from build123d import *

# Parameters (mm, degrees)
CROQUIS1_W              = 28
CROQUIS1_H              = 48
SALIENTE_EXTRUIR1_DEPTH = 2
CROQUIS2_R              = 1.25
CORTAR_EXTRUIR1_DEPTH   = 3
CROQUIS3_W              = 15
CROQUIS3_H              = 15
SALIENTE_EXTRUIR2_DEPTH = 6


with BuildPart() as part:
    # Croquis1 → Saliente-Extruir1 (new body)
    with BuildSketch(Plane.XY):
        Rectangle(CROQUIS1_W, CROQUIS1_H)
    extrude(amount=SALIENTE_EXTRUIR1_DEPTH)

    # Croquis2 → Cortar-Extruir1 (cut, through all)
    with BuildSketch(Plane.XY.offset(2)):
        with Locations((-10, 20)):
            Circle(CROQUIS2_R)
        with Locations((10, 20)):
            Circle(CROQUIS2_R)
        with Locations((10, -20)):
            Circle(CROQUIS2_R)
        with Locations((-10, -20)):
            Circle(CROQUIS2_R)
    extrude(amount=-CORTAR_EXTRUIR1_DEPTH, mode=Mode.SUBTRACT)

    # Croquis3 → Saliente-Extruir2 (add)
    with BuildSketch(Plane.XY.offset(2)):
        with Locations((6.5, 4.293122568)):
            Rectangle(CROQUIS3_W, CROQUIS3_H)
    extrude(amount=SALIENTE_EXTRUIR2_DEPTH)


solid = part.part
Can you work these out from the model? Positions are in its coordinate system, mm. A direction names the side the tool comes from. Give positions to 0.01 mm unless a question says otherwise; leave off trailing zeros. Write each loop counter-clockwise with the first axis right and the second up, starting at its lowest first coordinate (ties: lowest second). Pieces come first, ordered by that corner, then holes. Notation, with made-up numbers: (34, 25) -> (82, 25) arc R15 ccw to (82, 29) -> close; hole circle Ø10 at (19, 7). An arc over 180 degrees is marked (long way). Answer as a JSON object with one key per item and string values. Group by question number.
Item 1: Suppose I cut it at D-D (x = 10). Please give me the cut outline in (y, z).
Item 2: We'd pull the mould along Y, two halves only. Please class faces 1 (the face through (0, -24, 1)), 2 (the face through (6, 11.793, 5)), 3 (the face through (-10.99, 19.24, 1.01)): +Y half, -Y half, draft (parallel to the pull), parting line (faces both ways), or undercut.
Item 3: Suppose I cut it at B-B (y = 20). Please give me the cut outline in (x, z), plus the area to 3 significant figures.
Item 4: For faces 4 (the face through (9.01, 19.24, 1.01)), 5 (the face through (6, -3.207, 5)), 6 (the face through (-1, 4, 5)), which set-ups out of +Z, -Z, +X, -X, +Y, -Y let a thin tool reach every point of the face, with its end or its side?
Item 5: Suppose I cut it at A-A (x = -10). Please give me the cut outline in (y, z).
Item 6: I'm going to push flat-ended pins straight in: P1, Ø5, axis at x = -5.5, y = -18, coming from the +Z side; P2, Ø3, axis at y = 4, z = 6, coming from the -X side; P3, Ø3, axis at x = 9, z = 4.5, coming from the +Y side; P4, Ø2, axis at x = 10, y = -20, coming from the +Z side. Where does each tip first touch, or does it pass through?
Item 7: Please list where these lines run through material, in increasing order: line 1 (Y direction, x = -10, z = 1.5); line 2 (Z direction, x = -6, y = 11); line 3 (Y direction, x = 11, z = 4.5). Write a range as [from, to].
Item 8: Suppose I cut it at C-C (x = 4.25). Please give me the cut outline in (y, z).
Findings:
{
 "1": {"outline": "(-24, 0) -> (-21.25, 0) -> (-21.25, 2) -> (-24, 2) -> close; (-18.75, 0) -> (18.75, 0) -> (18.75, 2) -> (11.79, 2) -> (11.79, 8) -> (-3.21, 8) -> (-3.21, 2) -> (-18.75, 2) -> close; (21.25, 0) -> (24, 0) -> (24, 2) -> (21.25, 2) -> close"},
 "2": {"face 1": "-Y half", "face 2": "+Y half", "face 3": "undercut"},
 "3": {"outline": "(-14, 0) -> (-11.25, 0) -> (-11.25, 2) -> (-14, 2) -> close; (-8.75, 0) -> (8.75, 0) -> (8.75, 2) -> (-8.75, 2) -> close; (11.25, 0) -> (14, 0) -> (14, 2) -> (11.25, 2) -> close", "area": "46.0 mm²"},
 "4": {"face 4": "+Z, -Z", "face 5": "+Z, +X, -X, -Y", "face 6": "+Z, -X, +Y, -Y"},
 "5": {"outline": "(-24, 0) -> (-21.25, 0) -> (-21.25, 2) -> (-24, 2) -> close; (-18.75, 0) -> (18.75, 0) -> (18.75, 2) -> (-18.75, 2) -> close; (21.25, 0) -> (24, 0) -> (24, 2) -> (21.25, 2) -> close"},
 "6": {"P1": "stops at z = 2", "P2": "stops at x = -1", "P3": "stops at y = 11.79", "P4": "passes through"},
 "7": {"line 1": "y = [-24, -21.25], [-18.75, 18.75], [21.25, 24]", "line 2": "z = [0, 2]", "line 3": "y = [-3.21, 11.79]"},
 "8": {"outline": "(-24, 0) -> (24, 0) -> (24, 2) -> (11.79, 2) -> (11.79, 8) -> (-3.21, 8) -> (-3.21, 2) -> (-24, 2) -> close"}
}
